Part model, mm, in its own coordinate system. A direction names the side the tool comes from. Coordinates: 2 decimals unless noted, no trailing zeros. Write each loop counter-clockwise with the first axis right and the second up, starting at its lowest first coordinate (ties: lowest second). Pieces come first, ordered by that corner, then holes. Notation, with made-up numbers: (63, 6.5) - (100, 6.5) arc R22 cw to (100, 29.5) - close; hole circle Ø1 at (-17.75, -31). An arc over 180 degrees is marked (long way). Use a Markdown table: item, result.
```python
from build123d import *

# Parameters (mm, degrees)
F0_W      = 29
F0_H      = 16.5
F1_DEPTH  = 38.5
F2_T      = -2
F3_DEPTH  = 2.25
F4_SIZE   = 2
F5_SIZE   = 2
F6_SIZE   = 0.99999
F8_DEPTH  = 16.501
F9_W      = 12.5
F9_H      = 0.99999
F10_DEPTH = 2
F11_R     = 2
F12_DEPTH = 2.001
F13_W     = 7.54
F13_H     = 7.25
F13_R     = 1.1
F14_DEPTH = 4.35
F15_W     = 5.538
F15_H     = 5.533
F17_W     = 5.481
F17_H     = 4.583


# Not quite as in the source:
# - a fillet or chamfer is up to 0.001 mm smaller than in the source, because OpenCascade refuses the exact size


with BuildPart() as f1:
    # F0 (on Top) → F1 (new body)
    with BuildSketch(Plane.XY):
        with Locations((14.5, 8.25)):
            Rectangle(F0_W, F0_H)
    extrude(amount=F1_DEPTH)

    # F2
    f2_openings = [f1.faces().sort_by_distance(p)[0] for p in [
        (14.5, 8.25, 38.5),
    ]]
    offset(amount=F2_T, openings=f2_openings)

    # F3 (add): a face of the model
    f3_faces = [f1.faces().sort_by_distance(p)[0] for p in [
        (14.5, 8.25, 2),
    ]]
    extrude(f3_faces, amount=F3_DEPTH)

    # F4
    f4_edges = [f1.edges().sort_by_distance(p)[0] for p in [
        (0, 0, 19.25),
        (29, 0, 19.25),
        (29, 16.5, 19.25),
        (0, 16.5, 19.25),
    ]]
    chamfer(f4_edges, length=F4_SIZE)

    # F5 (call 1 of 4: OpenCascade refuses the feature's edges together)
    f5_edges = [f1.edges().sort_by_distance(p)[0] for p in [
        (14.5, 0, 0),
    ]]
    chamfer(f5_edges, length=F5_SIZE)

    # F5#2 (call 2 of 4)
    f5_2_edges = [f1.edges().sort_by_distance(p)[0] for p in [
        (0, 8.25, 0),
    ]]
    chamfer(f5_2_edges, length=F5_SIZE)

    # F5#3 (call 3 of 4)
    f5_3_edges = [f1.edges().sort_by_distance(p)[0] for p in [
        (14.5, 16.5, 0),
    ]]
    chamfer(f5_3_edges, length=F5_SIZE)

    # F5#4 (call 4 of 4)
    f5_4_edges = [f1.edges().sort_by_distance(p)[0] for p in [
        (29, 8.25, 0),
    ]]
    chamfer(f5_4_edges, length=F5_SIZE)

    # F6 (size 1 in the source; OpenCascade refuses exactly that, so slightly less here)
    f6_edges = [f1.edges().sort_by_distance(p)[0] for p in [
        (0, 8.25, 38.5),
        (14.5, 16.5, 38.5),
        (29, 8.25, 38.5),
        (14.5, 0, 38.5),
    ]]
    chamfer(f6_edges, length=F6_SIZE)

    # F7 (on face) → F8 (cut, through all)
    with BuildSketch(Plane.XZ):
        Polygon((6.464, 8.664), (6.464, 4.94), (23.536, 4.94), (23.536, 8.664), (17.364, 12.834), (12.635, 12.834), align=None)
    extrude(amount=-F8_DEPTH, mode=Mode.SUBTRACT)

    # F9 (on face) → F10 (cut, through all)
    with BuildSketch(Plane.YZ.offset(29)):
        with BuildLine():
            ThreePointArc((5.0038961688, 23.1590909091), (8.25, 22.25), (11.4961038312, 23.1590909091))
            ThreePointArc((11.4961038312, 23.1590909091), (8.25, 26.25), (5.0038961688, 23.1590909091))
        make_face()
        with BuildLine():
            ThreePointArc((5.0038961688, 23.1590909091), (8.1704306945, 19.7509741882), (11.5, 23))
            ThreePointArc((11.5, 23), (11.4990258118, 23.0795693055), (11.4961038312, 23.1590909091))
            ThreePointArc((11.4961038312, 23.1590909091), (8.25, 22.25), (5.0038961688, 23.1590909091))
        make_face()
        with BuildLine():
            ThreePointArc((5.0038961688, 23.1590909091), (8.25, 26.25), (11.4961038312, 23.1590909091))
            ThreePointArc((11.4961038312, 23.1590909091), (13.6975062618, 25.4361502113), (14.5, 28.5))
            Line((14.5, 28.5), (2, 28.5))
            ThreePointArc((2, 28.5), (2.8024937382, 25.4361502113), (5.0038961688, 23.1590909091))
        make_face()
        with BuildLine():
            Line((2, 28.5), (14.5, 28.5))
            ThreePointArc((14.5, 28.5), (8.25, 34.75), (2, 28.5))
        make_face()
        with BuildLine():
            ThreePointArc((2, 28.5), (8.25, 34.75), (14.5, 28.5))
            Line((14.5, 28.5), (14.5, 37.50001))
            Line((14.5, 37.50001), (2, 37.50001))
            Line((2, 37.50001), (2, 28.5))
        make_face()
        with Locations((8.25, 38.000005)):
            Rectangle(F9_W, F9_H)
    extrude(amount=-F10_DEPTH, mode=Mode.SUBTRACT)

    # F11 (on face) → F12 (cut, through all)
    with BuildSketch(Plane.YZ.offset(2)):
        with Locations((8.25, 23)):
            Circle(F11_R)
    extrude(amount=-F12_DEPTH, mode=Mode.SUBTRACT)

    # F13 (on face) → F14 (join)
    with BuildSketch(Plane(origin=(27, 0, 0), x_dir=(0, -1, 0), z_dir=(-1, 0, 0))):
        with Locations((-8.25, 7.875)):
            Rectangle(F13_W, F13_H)
        with Locations((-8.25, 9)):
            Circle(F13_R, mode=Mode.SUBTRACT)
    extrude(amount=F14_DEPTH)

    # F15 (on face) → F18 section 0
    with BuildSketch(Plane.YZ.offset(29)):
        with Locations((8.25, 8.0385)):
            Rectangle(F15_W, F15_H)
    # F17 (on offset) → F18 section 1
    with BuildSketch(Plane.YZ.offset(24.55)):
        with Locations((8.2215, 8.5135)):
            Rectangle(F17_W, F17_H)
    loft(mode=Mode.SUBTRACT)


solid = f1.part
```
Item 1: Band-saw the part on A-A, the plane y = 8.25. Count the separate pieces of the cut face and the enclosed holes in it, then the cut area to 3 significant figures.
From the geometry:
| item | result |
|---|---|
| separate pieces | 3 |
| enclosed holes | 0 |
| area | 215 mm^2 |
Item 2: Drop flat-ended pins along their axis: P1, Ø1, axis at y = 16, z = 7, coming from the -X side; P2, Ø2, axis at x = 24.5, y = 9.5, coming from the +Z side; P3, Ø5, axis at y = 8.25, z = 23, coming from the +X side. Give the stop position or say it passes through.
From the geometry:
| item | result |
|---|---|
| P1 | x = 1 |
| P2 | z = 11.5 |
| P3 | x = 2 |
Item 3: Drill centre lines: probe 1 along Y at (x, z) = (23.1, 9); probe 2 along Z at (x, y) = (23.7, 8.25); probe 3 along Y at (x, z) = (26, 30.5). Where is each one in solid material? Low to high.
From the geometry:
| item | result |
|---|---|
| probe 1 | 0 to 2, 4.48 to 7.15, 9.35 to 12.02, 14.5 to 16.5 |
| probe 2 | 0 to 7.9, 10.1 to 11.5 |
| probe 3 | 0 to 2, 14.5 to 16.5 |
Item 4: Band-saw the part on C-C, the plane y = 13. Give the cut face in (x, z), then the cut area to 3 significant figures.
From the geometry:
| item | result |
|---|---|
| outline | (0, 2) - (2, 0) - (27, 0) - (29, 2) - (29, 24.44) - (27, 24.44) - (27, 4.25) - (2, 4.25) - (2, 38.5) - (1, 38.5) - (0, 37.5) - close |
| area | 228 mm^2 |
Item 5: Two-plate mould, pull along Y, no slides. Class faces 1 (the face through (15, 1, 4.94)), 2 (the face through (25, 8, 11.5)), 3 (the face through (28, 1, 19)): pulls with the +Y half, pulls with the -Y half, needs draft (parallel to the pull), parting line crosses it, or undercut.
From the geometry:
| item | result |
|---|---|
| face 1 | needs draft |
| face 2 | undercut |
| face 3 | pulls with the -Y half |
Item 6: Which spindle directions (+Z, -Z, +X, -X, +Y, -Y) get a long thin tool onto all of the face, cutting with end or side? Do faces 4 (the face through (2, 10, 21)), 5 (the face through (6.464, 1, 7)), 6 (the face through (28.01, 2.78, 25.48)), 7 (the face through (23.613, 7.234, 8.579)), 8 (the face through (1, 8, 1)). Say none if no direction does.
From the geometry:
| item | result |
|---|---|
| face 4 | +Z |
| face 5 | +Y, -Y |
| face 6 | +Z, +X |
| face 7 | +X |
| face 8 | -Z, -X, +Y, -Y |
Item 7: Band-saw the part on B-B, the plane x = 8.75. Give the cut face in (y, z), then the cut area to 3 significant figures.
From the geometry:
| item | result |
|---|---|
| outline | (0, 2) - (2, 0) - (14.5, 0) - (16.5, 2) - (16.5, 4.94) - (14.5, 4.94) - (14.5, 4.25) - (2, 4.25) - (2, 4.94) - (0, 4.94) - close; (0, 10.21) - (2, 10.21) - (2, 38.5) - (1, 38.5) - (0, 37.5) - close; (14.5, 10.21) - (16.5, 10.21) - (16.5, 37.5) - (15.5, 38.5) - (14.5, 38.5) - close |
| area | 181 mm^2 |
